Autodesk Inventor part; units mm, degrees
ref_plane "YZ Plane" through (0, 0, 0) normal (1, 0, 0) x (0, 1, 0)
ref_plane "XZ Plane" through (0, 0, 0) normal (0, 1, 0) x (-1, 0, 0)
ref_plane "XY Plane" through (0, 0, 0) normal (0, 0, 1) x (1, 0, 0)
sketch "スケッチ1" plane through (0, 0, 0) normal (0, 1, 0) x (-1, 0, 0)
  line L0 (130, 81) -> (-130, 81)
  line L1 (-130, 81) -> (-130, -81)
  line L2 (-130, -81) -> (130, -81)
  line L3 (130, -81) -> (130, 81)
  line L4 (130, 81) -> (-130, -81) construction
  line L5 (-130, 81) -> (130, -81) construction
  point P0 (0, 0)
  dimension "d0" = 260
  dimension "d1" = 162
extrude "押し出し1" add sketch "スケッチ1" along normal blind 3
sketch "スケッチ7" plane through (0, 3, 0) normal (0, 1, 0) x (1, 0, 0)
  line L0 (-130, 81) -> (-130, -81)
  line L1 (130, -81) -> (130, 81)
  line L2 (130, 81) -> (-130, 81)
  point P0 (0, 0)
  point P1 (-116, 67)
  point P2 (112, 67)
  point P3 (112, -63)
  point P4 (-116, -63)
  dimension "d23" = 14
  dimension "d25" = 130
  dimension "d26" = 130
  dimension "d27" = 14
  dimension "d29" = 14
  dimension "d38" = 228
  dimension "d39" = 228
  dimension "d40" = 14
hole "穴1" at (-116, 3, -67) at (112, 3, -67) at (112, 3, 63) at (-116, 3, 63) direction (0, -1, 0) diameter 3.2 depth 8
sketch "スケッチ8" plane through (0, 3, 0) normal (0, 1, 0) x (1, 0, 0)
  line L0 (130, 81) -> (-130, 81)
  line L1 (-130, 81) -> (126, 81)
  line L2 (126, 81) -> (126, -77)
  line L3 (126, -77) -> (-130, -77)
  line L4 (-130, -77) -> (-130, 81)
  circle A0 centre (-116, 67) radius 1.6
  circle A1 centre (112, 67) radius 1.6
  circle A2 centre (-116, -63) radius 1.6
  circle A3 centre (-116, -63) radius 1.6
  circle A4 centre (112, -63) radius 1.6
  circle A5 centre (112, 67) radius 1.6
  circle A6 centre (-116, 67) radius 1.6
  line L5 (130, -81) -> (130, 81)
  line L6 (130, 81) -> (-130, 81)
  line L7 (-130, 81) -> (-130, -81)
  line L8 (-130, -81) -> (130, -81)
  point P0 (0, 0)
  dimension "d41" = 14
  dimension "d42" = 14
  dimension "d43" = 14
extrude "押し出し4" cut sketch "スケッチ8" against normal blind 10 contours L5 L8 L7 L3 L2 L0
fillet "フィレット1" radius 5 4 edges at (-130, 1.5, -81) (-130, 1.5, 77) (126, 1.5, -81) (126, 1.5, 77)
sketch "スケッチ9" plane through (0, 3, 0) normal (0, 1, 0) x (1, 0, 0)
  arc A0 (121, -77) -> (126, -72) centre (121, -72) ccw
  line L0 (126, -72) -> (126, 76)
  arc A1 (126, 76) -> (121, 81) centre (121, 76) ccw
  line L1 (121, 81) -> (-125, 81)
  arc A2 (-125, 81) -> (-130, 76) centre (-125, 76) ccw
  line L2 (-130, 76) -> (-130, -72)
  arc A3 (-130, -72) -> (-125, -77) centre (-125, -72) ccw
  line L3 (-125, -77) -> (121, -77)
  circle A4 centre (-116, 67) radius 1.6
  circle A5 centre (112, 67) radius 1.6
  circle A6 centre (112, -63) radius 1.6
  circle A7 centre (-116, -63) radius 1.6
  circle A8 centre (-116, 67) radius 3
  circle A9 centre (-116, -63) radius 3
  circle A10 centre (112, -63) radius 3
  circle A11 centre (112, 67) radius 3
  point P0 (0, 0)
  dimension "d47" = 6
  dimension "d48" = 6
  dimension "d49" = 6
  dimension "d50" = 6
extrude "押し出し5" cut sketch "スケッチ9" against normal blind 2 contours A4 | A5 | A6 | A7 | A8 | A9 | A10 | A11
sketch "スケッチ10" plane through (0, 3, 0) normal (0, 1, 0) x (1, 0, 0)
  line L0 (121, 81) -> (-125, 81)
  line L1 (121, -77) -> (-125, -77)
  line L2 (-90, 81) -> (-69.8, 81)
  line L3 (-69.8, 81) -> (-69.8, -77)
  line L4 (-69.8, -77) -> (-90, -77)
  line L5 (-90, -77) -> (-90, 81)
  line L6 (86, 81) -> (65.8, 81)
  line L7 (65.8, 81) -> (65.8, -77)
  line L8 (65.8, -77) -> (86, -77)
  line L9 (86, -77) -> (86, 81)
  line L10 (-69.8, 81) -> (-49.6, 81)
  line L11 (-49.6, 81) -> (-49.6, -77)
  line L12 (-49.6, -77) -> (-69.8, -77)
  line L13 (-69.8, -77) -> (-69.8, 81)
  line L14 (65.8, 81) -> (45.6, 81)
  line L15 (45.6, 81) -> (45.6, -77)
  line L16 (45.6, -77) -> (65.8, -77)
  line L17 (65.8, -77) -> (65.8, 81)
  line L18 (45.6, -77) -> (25.4, -77)
  line L19 (25.4, -77) -> (25.4, 81)
  line L20 (25.4, 81) -> (45.6, 81)
  line L21 (45.6, 81) -> (45.6, -77)
  line L22 (-49.6, 81) -> (-29.4, 81)
  line L23 (-29.4, 81) -> (-29.4, -77)
  line L24 (-29.4, -77) -> (-49.6, -77)
  line L25 (-49.6, -77) -> (-49.6, 81)
  line L26 (-130, 76) -> (-130, -72)
  line L27 (126, -72) -> (126, 76)
  line L28 (-69.7, 81) -> (-49.7, 81)
  line L29 (-49.7, 81) -> (-49.7, -77)
  line L30 (-49.7, -77) -> (-69.7, -77)
  line L31 (-69.7, -77) -> (-69.7, 81)
  line L32 (0, 0) -> (0, 23.1289)
  line L33 (-69.9, 81) -> (-87.9535, 81)
  line L34 (-87.9535, 81) -> (-87.9535, -77)
  line L35 (-87.9535, -77) -> (-69.9, -77)
  line L36 (-69.9, -77) -> (-69.9, 81)
  point P0 (-59.8, 61)
  point P1 (-59.8, -57)
  point P2 (55.8, 61)
  point P3 (55.8, -57)
  dimension "d53" = 20.2
  dimension "d54" = 20.2
  dimension "d55" = 20.2
  dimension "d56" = 20.2
  dimension "d57" = 20.2
  dimension "d58" = 20.2
  dimension "d59" = 40
  dimension "d60" = 40
  dimension "d61" = 0.1
  dimension "d62" = 0.1
  dimension "d63" = 20
  dimension "d64" = 20
  dimension "d66" = 256
  dimension "d67" = 158
  dimension "d68" = 0.2
  dimension "d69" = 20
  dimension "d70" = 118
  dimension "d71" = 70.2
  dimension "d72" = 70.2
  dimension "d80" = 70.2
  dimension "d81" = 70.2
  dimension "d14" = 30
  dimension "d15" = 30
  dimension "d16" = 30
  dimension "d17" = 30
hole "穴2" at (-59.8, 3, -61) at (-59.8, 3, 57) at (55.8, 3, -61) at (55.8, 3, 57) direction (0, -1, 0) diameter 3.2 depth 8
equation "\"d42\" = d41"
equation "\"d43\" = d41"
equation "\"d48\" = d47"
equation "\"d49\" = d47"
equation "\"d50\" = d47"
equation "\"d54\" = d53"
equation "\"d55\" = d53"
equation "\"d56\" = d54"
equation "\"d57\" = d56"
equation "\"d58\" = d57"
equation "\"d62\" = d61"
properties part number "BP_BOX-Above" material "アセタール樹脂、白"
Read the model definition and answer for the solid it produces. Units are mm, in the model's axes. A direction names the side the tool comes from. Round coordinates to 2 decimals unless told otherwise and drop trailing zeros.
1. Straight lines are drawn through the part: L1, parallel to Z at x = 56, y = 1.85; L2, parallel to X at y = 0.3, z = -67; L3, parallel to Z at x = -61, y = 2.15. For each, find the intervals that lie inside material, in ascending order.
2. Which of the six approach directions +Z, -Z, +X, -X, +Y, -Y give full straight-line access (tool end or side, diameter ignored) to faces 4 (the face through (-128, 1, 76)), 5 (the face through (114.86, 2.01, 62.1))?
3. Determine the mould class of faces 1 (the face through (113.3, 1, -65.7)), 2 (the face through (125, 1, 75)), 3 (the face through (124, 1, -80)) for opening direction Z: pulls with the +Z half, pulls with the -Z half, needs draft (parallel to the pull), parting line crosses it, or undercut.
4. Given pin 1 Ø2.5 at (x, z) = (-116, -67) entering from +Y; pin 2 Ø3 at (x, z) = (-115, 64) entering from +Y, each flat-ended and moving along its own axis, determine where each tip first touches the part or whether it passes through.
Values:
1. L1: z = -81 to -62.59, -59.41 to 55.41, 58.59 to 77
1. L2: x = -130 to -117.6, -114.4 to 110.4, 113.6 to 126
1. L3: z = -81 to -62.06, -59.94 to 55.94, 58.06 to 77
2. face 4: +Z, -X, +Y, -Y
2. face 5: +Y
3. face 1: undercut
3. face 2: pulls with the +Z half
3. face 3: pulls with the -Z half
4. pin 1: passes through
4. pin 2: stops at y = 1
